Work out the finished part from the listing and answer in its coordinate system (mm). Face numbers are marked on the shaded views. Coordinates: 2 decimals unless noted, no trailing zeros. Write each loop counter-clockwise with the first axis right and the second up, starting at its lowest first coordinate (ties: lowest second). Pieces come first, ordered by that corner, then holes. Notation, with made-up numbers: (70.5, 14) - (88.5, 14) arc R11 cw to (88.5, 25) - close; hole circle Ø3 at (-34, 61.25). An arc over 180 degrees is marked (long way). Use a Markdown table: item, result. Add a question column.
(1) Given pin 1 Ø11 at (y, z) = (-6.5, 135.5) entering from +X; pin 2 Ø3 at (x, z) = (20.5, 37) entering from -Y; pin 3 Ø2 at (y, z) = (-20, 161.5) entering from +X, each flat-ended and moving along its own axis, determine where each tip first touches the part or whether it passes through.
(2) The part is cut by section B-B, the plane z = 107.5. Give the vertices of the cut face in (x, y), then the cut area to 3 significant figures.
(3) The part is cut by section D-D, the plane y = -8. Give the vertices of the cut face in (x, z).
(4) For a pull along Y with two mould halves and no side action, classify the marked faces 1, 2, 3 and 4 as released by +Y, released by -Y, zero draft, split by the parting line, or undercut.
(5) Find the intervals of material crossed by line 1 (X direction, y = 4, z = 139); line 2 (Y direction, x = 33, z = 174); line 3 (Y direction, x = 23.5, z = 66), in increasing order. Write a range as from..to.
Autodesk Inventor part; units mm, degrees
ref_plane "Начальная плоскость" through (0, 0, 0) normal (0, 0, 1) x (1, 0, 0)
ref_plane "Конечная плоскость" through (0, 0, 226.4162) normal (0, 0, 1) x (1, 0, 0)
ref_plane "РабПлоскость8" through (36, 423.958, 290.4468) normal (0, 0.5652, -0.825) x (1, 0, 0)
ref_plane "Начальная плоскость" through (0, 0, 0) normal (0, 0, 1) x (1, 0, 0)
ref_plane "Конечная плоскость" through (0, 0, 226.4162) normal (0, 0, 1) x (1, 0, 0)
sketch "Эскиз" plane through (0, 0, 0) normal (0, 0, 1) x (1, 0, 0)
  line L0 (36, -32.5) -> (0, -32.5)
  line L1 (36, -32.5) -> (36, -28.696)
  line L2 (33.6994, -26.2039) -> (9.9215, -24.3017)
  line L3 (4.4, -18.3208) -> (4.4, 18.3208)
  line L4 (33.6994, 26.2039) -> (9.9215, 24.3017)
  line L5 (36, 28.696) -> (36, 32.5)
  line L6 (0, 32.5) -> (36, 32.5)
  line L7 (0, -32.5) -> (0, 32.5)
  arc A0 (4.4, -18.3208) -> (9.9215, -24.3017) centre (10.4, -18.3208) ccw
  arc A1 (9.9215, 24.3017) -> (4.4, 18.3208) centre (10.4, 18.3208) ccw
  arc A2 (36, -28.696) -> (33.6994, -26.2039) centre (33.5, -28.696) ccw
  arc A3 (33.6994, 26.2039) -> (36, 28.696) centre (33.5, 28.696) ccw
  line L8 (0, 45.5) -> (0, -45.5) construction
  line L9 (-7.2974, 0) -> (43.7847, 0) construction
  point P0 (36, -26.388)
  point P1 (4.4, -23.86)
  point P2 (4.4, 23.86)
  point P3 (36, 26.388)
  dimension "d3" = 36
  dimension "d5" = 4.4
  dimension "d7" = 65
  dimension "d9" = 8.64
  dimension "d11" = 8.64
  dimension "d13" = 6.112
  dimension "d15" = 6.112
  dimension "d22" = 6
  dimension "d23" = 2.5
  dimension "d24" = 32.5
  dimension "d25" = 0
extrude "Тело" add sketch "Эскиз" along normal up to surface (226.4162 mm away) from surface at 0
sketch "Sketch3" plane through (0, 0, 0) normal (0, 0, 1) x (1, 0, 0)
  line L0 (0, 0) -> (10, 0)
ref_plane "Work Plane7" through (0, 0, 0) normal (0, -1, 0) x (1, 0, 0)
sketch "Sketch4" plane through (0, 0, 0) normal (0, -1, 0) x (1, 0, 0)
  line L0 (-2, 0) -> (12, 0)
  line L1 (-2, 226.4162) -> (12, 226.4162)
  dimension "d29" = 226.4162
ref_plane "РабПлоскость8" through (36, 423.958, 290.4468) normal (0, 0.5652, -0.825) x (1, 0, 0)
split "Разделение1" plane through (36, 423.958, 290.4468) removes the side toward (0, 0.5652, -0.825)
ref_plane "РабПлоскость9" through (36, -65.6795, 158.7646) normal (0, -0.5674, 0.8234) x (1, 0, 0)
split "Разделение2" plane through (36, -65.6795, 158.7646) removes the side toward (0, -0.5674, 0.8234)
ref_plane "РабПлоскость10" through (-29, -95.3234, 138.3382) normal (0, -0.8234, -0.5674) x (1, 0, 0)
split "Разделение3" plane through (-29, -95.3234, 138.3382) removes the side toward (0, -0.8234, -0.5674)
equation "\"d3\" = b"
equation "\"d7\" = ParH"
equation "\"d22\" = R"
equation "\"d23\" = R1"
equation "\"d24\" = 0.5 * d7"
equation "\"d16\" = G_L"
equation "\"R1\" = 2.5"
equation "\"R\" = 6"
equation "\"t1\" = 4.4"
equation "\"t2\" = 7.2"
equation "\"ParH\" = 65"
equation "\"b\" = 36"
equation "\"msp_x1\" = 0.04 * b"
equation "\"msp_x2\" = -0.08 * t1 + 0.04 * b"
equation "\"G_L\" = d29"
equation "\"ex\" = 0"
equation "\"G_OFFSET_START\" = 0"
equation "\"G_OFFSET_END\" = 22.18382"
equation "\"d27\" = G_OFFSET_END + B_L"
equation "\"B_L\" = 204.2324"
properties part number "Швеллер 6.5U-226,42 ГОСТ 8240-97" material "Сталь, мягкая"
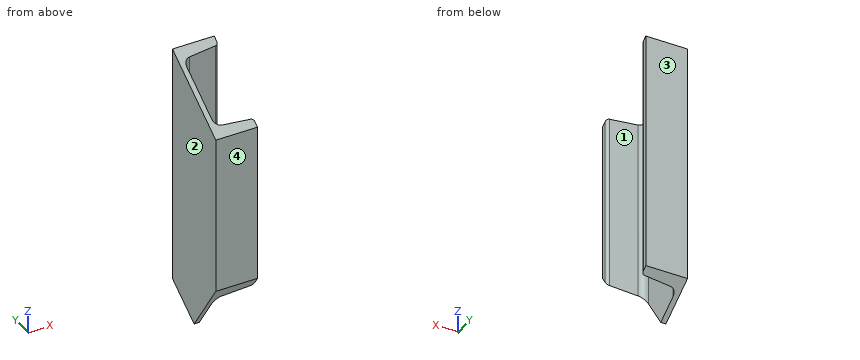
Model answer:
| question | item | result |
|---|---|---|
| 1 | pin 1 | x = 4.4 |
| 1 | pin 2 | y = -26.53 |
| 1 | pin 3 | x = 5.03 |
| 2 | outline | (0, -32.5) - (36, -32.5) - (36, -28.7) arc R2.5 ccw to (33.7, -26.2) - (9.92, -24.3) arc R6 cw to (4.4, -18.32) - (4.4, 18.32) arc R6 cw to (9.92, 24.3) - (33.7, 26.2) arc R2.5 ccw to (36, 28.7) - (36, 32.5) - (0, 32.5) - close |
| 2 | area | 763 mm^2 |
| 3 | outline | (0, 11.62) - (4.4, 11.62) - (4.4, 198.51) - (0, 198.51) - close |
| 4 | face 1 | undercut |
| 4 | face 2 | zero draft |
| 4 | face 3 | released by +Y |
| 4 | face 4 | released by -Y |
| 5 | line 1 | 0..4.4 |
| 5 | line 2 | -32.5..-26.15, 26.15..32.5 |
| 5 | line 3 | -32.5..-25.39, 25.39..32.5 |
